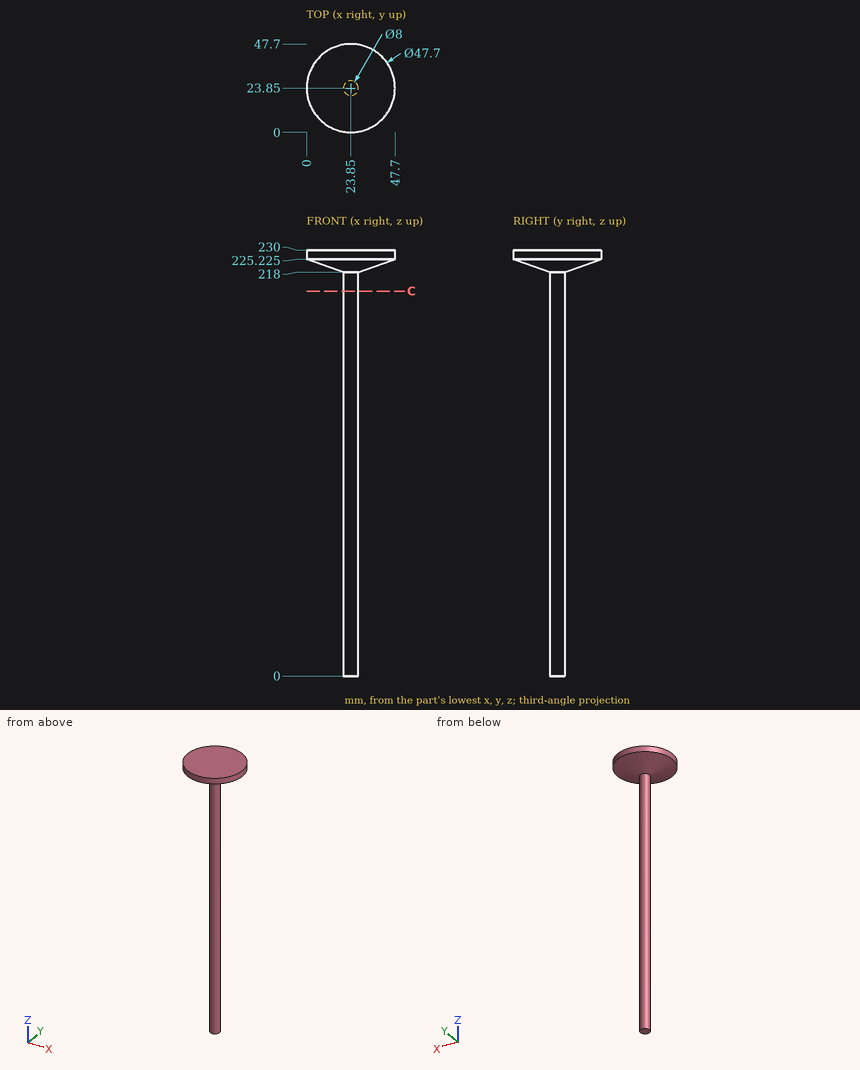
Drawing for the job (mm, zero at the part's lowest x, y, z). Round coordinates to 2 decimals unless told otherwise and drop trailing zeros. Loops run counter-clockwise (first coordinate to the right, second up) from the corner with the lowest first, then second, coordinate; pieces in that order, holes last. Notation, with made-up numbers: M 60,89.25 L 64,89.25 A9 cw 64,104.25 Z; hole C 9.5,-34.5 d11. An arc over 180 degrees is marked long. Use a Markdown table: item, result. Add a question column.
(1) Drill centre lines: line 1 (Z direction, x = 24.5, y = 34.5); line 2 (Z direction, x = 25, y = 18); line 3 (X direction, y = 26, z = 111.5). Where is each one in solid material? Low to high.
(2) Flat gauge pins, fed straight in: pin 1 (2 mm diameter, centred on y = 22.5, z = 136, fed in from -X); pin 2 (10 mm diameter, centred on y = 26, z = 68.5, fed in from +X); pin 3 (12 mm diameter, centred on x = 11.5, y = 29, fed in from -Z); pin 4 (10 mm diameter, centred on y = 13, z = 167, fed in from +X). Where does each tip first touch, or does it go through?
(3) Cut at C-C (z = 208). Give the cut face in (x, y).
Geometry says:
| question | item | result |
|---|---|---|
| 1 | line 1 | z = 220.43 to 230 |
| 1 | line 2 | z = 218.71 to 230 |
| 1 | line 3 | x = 20.48 to 27.22 |
| 2 | pin 1 | stops at x = 19.87 |
| 2 | pin 2 | stops at x = 27.85 |
| 2 | pin 3 | stops at z = 219.23 |
| 2 | pin 4 | passes through |
| 3 | outline | C 23.85,23.85 d8 |
